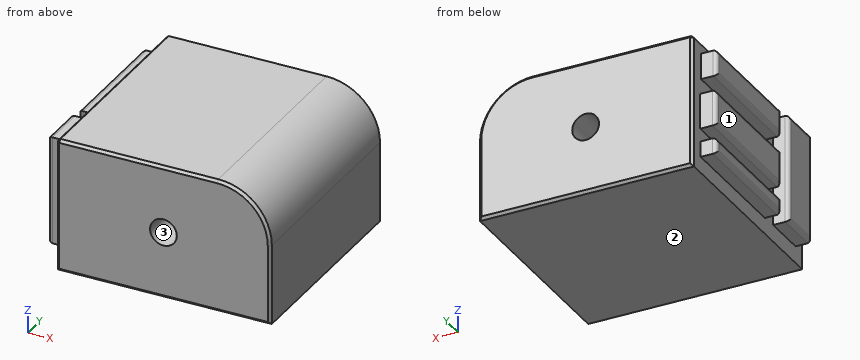
from build123d import *

# Parameters (mm, degrees)
F0_W     = 16
F0_H     = 16
F1_DEPTH = 10
F2_R     = 4
F3_W     = 9.202218
F3_H     = 1.946622
F3_W_2   = 9.320195
F3_H_2   = 2.654486
F3_W_3   = 9.261206
F3_H_3   = 1.179772
F3_W_4   = 3.244372
F3_H_4   = 8.081435
F4_DEPTH = 1.2
F5_R     = 0.3
F6_SIZE  = 0.2
F7_R     = 1
F8_DEPTH = 16.001


with BuildPart() as f1:
    # F0 (on Top) → F1 (new body)
    with BuildSketch(Plane.XY):
        Rectangle(F0_W, F0_H)
    extrude(amount=F1_DEPTH)

    # F2
    f2_edges = [f1.edges().sort_by_distance(p)[0] for p in [
        (8, 0, 10),
    ]]
    fillet(f2_edges, radius=F2_R)

    # F3 (on face) → F4 (join)
    with BuildSketch(Plane(origin=(-8, 0, 0), x_dir=(0, -1, 0), z_dir=(-1, 0, 0))):
        with Locations((-2.188604, 8.136063)):
            Rectangle(F3_W, F3_H)
        with Locations((-2.247592, 4.655737)):
            Rectangle(F3_W_2, F3_H_2)
        with Locations((-2.218098, 1.794791)):
            Rectangle(F3_W_3, F3_H_3)
        with Locations((5.214463, 5.304612)):
            Rectangle(F3_W_4, F3_H_4)
    extrude(amount=F4_DEPTH)

    # F5
    f5_edges = [f1.edges().sort_by_distance(p)[0] for p in [
        (-9.2, 2.188604, 9.109374),
        (-9.2, -2.412505, 8.136063),
        (-9.2, 2.188604, 7.162752),
        (-9.2, 2.247592, 5.98298),
        (-9.2, -2.412505, 4.655737),
        (-9.2, 2.247592, 3.328494),
        (-9.2, 2.218098, 2.384677),
        (-9.2, -2.412505, 1.794791),
        (-9.2, 2.218098, 1.204905),
        (-9.2, -5.214463, 9.345329),
        (-9.2, -6.836649, 5.304612),
        (-9.2, -3.592277, 5.304612),
        (-9.2, -5.214463, 1.263894),
        (-9.2, 6.789713, 8.136063),
        (-9.2, 6.90769, 4.655737),
        (-9.2, 6.848701, 1.794791),
    ]]
    fillet(f5_edges, radius=F5_R)

    # F6
    f6_edges = [f1.edges().sort_by_distance(p)[0] for p in [
        (8, -8, 3),
        (6.828427, -8, 8.828427),
        (0, -8, 0),
        (-2, -8, 10),
        (-8, -8, 5),
        (8, 8, 3),
        (6.828427, 8, 8.828427),
        (0, 8, 0),
        (-2, 8, 10),
        (-8, 8, 5),
        (-8, 0, 10),
    ]]
    chamfer(f6_edges, length=F6_SIZE)

    # F7 (on face) → F8 (cut, through all)
    with BuildSketch(Plane.XZ.offset(8)):
        with Locations((0, 5)):
            Circle(F7_R)
    extrude(amount=-F8_DEPTH, mode=Mode.SUBTRACT)


solid = f1.part
Could you check a few things on this model? Use its own coordinates, in mm. Face numbers are marked on the shaded views. Give positions to 0.01 mm unless a question says otherwise; leave off trailing zeros. Loops run counter-clockwise (first coordinate to the right, second up) from the corner with the lowest first, then second, coordinate; pieces in that order, holes last. Notation, with made-up numbers: M 65,-32 L 93,-32 A3 cw 93,-27 Z; hole C 18,-20 d2. An arc over 180 degrees is marked long. Answer as a JSON object with one key per item and string values.
Q1. If I drill on probe 1 along Y at (x, z) = (-8.5, 3.75); probe 2 along Z at (x, y) = (0, 4.25); probe 3 along X at (y, z) = (-6.5, 6.5), over which ranges is the centre line in solid material (lowest first)? Write a range as [from, to].
Values found:
{"probe 1": "y = [-6.84, -3.59], [-2.41, 6.91]", "probe 2": "z = [0, 4], [6, 10]", "probe 3": "x = [-9.2, 7.97]"}
Q2. Suppose I cut it at C-C, the plane y = 1.25. List the corners of the cut face in (x, z) for me.
Values found:
{"outline": "M -9.2,1.5 A0.3 ccw -8.9,1.2 L -8,1.2 L -8,0 L 8,0 L 8,6 A4 ccw 4,10 L -7.8,10 L -8,9.8 L -8,9.11 L -8.9,9.11 A0.3 ccw -9.2,8.81 L -9.2,7.46 A0.3 ccw -8.9,7.16 L -8,7.16 L -8,5.98 L -8.9,5.98 A0.3 ccw -9.2,5.68 L -9.2,3.63 A0.3 ccw -8.9,3.33 L -8,3.33 L -8,2.38 L -8.9,2.38 A0.3 ccw -9.2,2.08 Z; hole C 0,5 d2"}
Q3. Suppose I cut it at B-B, the plane x = 0. List the corners of the cut face in (y, z) for me, plus the area to 3 significant figures.
Values found:
{"outline": "M -8,0.2 L -7.8,0 L 7.8,0 L 8,0.2 L 8,4 L -8,4 Z; M -8,6 L 8,6 L 8,9.8 L 7.8,10 L -7.8,10 L -8,9.8 Z", "area": "128 mm²"}
Q4. If we mould it in two halves opening along Z, with no side actions, what happens to the marked faces 1, 2 and 3? For each: pulls with the +Z half, pulls with the -Z half, needs draft (parallel to the pull), parting line crosses it, or undercut.
Values found:
{"face 1": "needs draft", "face 2": "pulls with the -Z half", "face 3": "undercut"}
Q5. Suppose I cut it at D-D, the plane y = -3. List the corners of the cut face in (x, z) for me, plus the area to 3 significant figures.
Values found:
{"outline": "M -8,0 L 8,0 L 8,6 A4 ccw 4,10 L -7.8,10 L -8,9.8 Z; hole C 0,5 d2", "area": "153 mm²"}
Q6. Suppose I cut it at A-A, the plane z = 5. List the corners of the cut face in (x, y) for me.
Values found:
{"outline": "M -9.2,-6.54 A0.3 ccw -8.9,-6.84 L -8,-6.84 L -8,-7.8 L -7.8,-8 L -1,-8 L -1,8 L -7.8,8 L -8,7.8 L -8,6.91 L -8.9,6.91 A0.3 ccw -9.2,6.61 L -9.2,-2.11 A0.3 ccw -8.9,-2.41 L -8,-2.41 L -8,-3.59 L -8.9,-3.59 A0.3 ccw -9.2,-3.89 Z; M 1,-8 L 7.8,-8 L 8,-7.8 L 8,7.8 L 7.8,8 L 1,8 Z"}
Q7. For P1, Ø0.7, axis at x = -8.5, z = 5, coming from the -Y side; P2, Ø0.7, axis at x = -8.5, y = 3, coming from the -Z side, each with a flat end and sliding along its axis, tell me the tip position at first contact or that it passes through.
Values found:
{"P1": "stops at y = -6.84", "P2": "stops at z = 1.2"}
